```python
from build123d import *

# Parameters (mm, degrees)
SKETCH1_R           = 3.35
BOSS_EXTRUDE1_DEPTH = 300


with BuildPart() as part:
    # Sketch1 → Boss-Extrude1 (new body)
    with BuildSketch(Plane.XY):
        with BuildLine():
            Line((-9.853553391, -11.978553391), (-5.771446609, -7.896446609))
            ThreePointArc((-5.771446609, -7.896446609), (-5.609234935, -7.788060234), (-5.417893219, -7.75))
            Line((-5.417893219, -7.75), (5.417893219, -7.75))
            ThreePointArc((5.417893219, -7.75), (5.609234935, -7.788060234), (5.771446609, -7.896446609))
            Line((5.771446609, -7.896446609), (9.853553391, -11.978553391))
            ThreePointArc((9.853553391, -11.978553391), (9.961939766, -12.140765065), (10, -12.332106781))
            Line((10, -12.332106781), (10, -16))
            ThreePointArc((10, -16), (9.707106781, -16.707106781), (9, -17))
            Line((9, -17), (8, -17))
            ThreePointArc((8, -17), (7.292893219, -16.707106781), (7, -16))
            ThreePointArc((7, -16), (6.853553391, -15.646446609), (6.5, -15.5))
            Line((6.5, -15.5), (5, -15.5))
            ThreePointArc((5, -15.5), (4.292893219, -15.792893219), (4, -16.5))
            Line((4, -16.5), (4, -18.5))
            ThreePointArc((4, -18.5), (4.439339828, -19.560660172), (5.5, -20))
            Line((5.5, -20), (17, -20))
            ThreePointArc((17, -20), (19.121320344, -19.121320344), (20, -17))
            Line((20, -17), (20, -5.5))
            ThreePointArc((20, -5.5), (19.560660172, -4.439339828), (18.5, -4))
            Line((18.5, -4), (16.5, -4))
            ThreePointArc((16.5, -4), (15.792893219, -4.292893219), (15.5, -5))
            Line((15.5, -5), (15.5, -6.5))
            ThreePointArc((15.5, -6.5), (15.646446609, -6.853553391), (16, -7))
            ThreePointArc((16, -7), (16.707106781, -7.292893219), (17, -8))
            Line((17, -8), (17, -9))
            ThreePointArc((17, -9), (16.707106781, -9.707106781), (16, -10))
            Line((16, -10), (12.332106781, -10))
            ThreePointArc((12.332106781, -10), (12.140765065, -9.961939766), (11.978553391, -9.853553391))
            Line((11.978553391, -9.853553391), (7.896446609, -5.771446609))
            ThreePointArc((7.896446609, -5.771446609), (7.788060234, -5.609234935), (7.75, -5.417893219))
            Line((7.75, -5.417893219), (7.75, 5.417893219))
            ThreePointArc((7.75, 5.417893219), (7.788060234, 5.609234935), (7.896446609, 5.771446609))
            Line((7.896446609, 5.771446609), (11.978553391, 9.853553391))
            ThreePointArc((11.978553391, 9.853553391), (12.140765065, 9.961939766), (12.332106781, 10))
            Line((12.332106781, 10), (16, 10))
            ThreePointArc((16, 10), (16.707106781, 9.707106781), (17, 9))
            Line((17, 9), (17, 8))
            ThreePointArc((17, 8), (16.707106781, 7.292893219), (16, 7))
            ThreePointArc((16, 7), (15.646446609, 6.853553391), (15.5, 6.5))
            Line((15.5, 6.5), (15.5, 5))
            ThreePointArc((15.5, 5), (15.792893219, 4.292893219), (16.5, 4))
            Line((16.5, 4), (18.5, 4))
            ThreePointArc((18.5, 4), (19.560660172, 4.439339828), (20, 5.5))
            Line((20, 5.5), (20, 17))
            ThreePointArc((20, 17), (19.121320344, 19.121320344), (17, 20))
            Line((17, 20), (5.5, 20))
            ThreePointArc((5.5, 20), (4.439339828, 19.560660172), (4, 18.5))
            Line((4, 18.5), (4, 16.5))
            ThreePointArc((4, 16.5), (4.292893219, 15.792893219), (5, 15.5))
            Line((5, 15.5), (6.5, 15.5))
            ThreePointArc((6.5, 15.5), (6.853553391, 15.646446609), (7, 16))
            ThreePointArc((7, 16), (7.292893219, 16.707106781), (8, 17))
            Line((8, 17), (9, 17))
            ThreePointArc((9, 17), (9.707106781, 16.707106781), (10, 16))
            Line((10, 16), (10, 12.332106781))
            ThreePointArc((10, 12.332106781), (9.961939766, 12.140765065), (9.853553391, 11.978553391))
            Line((9.853553391, 11.978553391), (5.771446609, 7.896446609))
            ThreePointArc((5.771446609, 7.896446609), (5.609234935, 7.788060234), (5.417893219, 7.75))
            Line((5.417893219, 7.75), (-5.417893219, 7.75))
            ThreePointArc((-5.417893219, 7.75), (-5.609234935, 7.788060234), (-5.771446609, 7.896446609))
            Line((-5.771446609, 7.896446609), (-9.853553391, 11.978553391))
            ThreePointArc((-9.853553391, 11.978553391), (-9.961939766, 12.140765065), (-10, 12.332106781))
            Line((-10, 12.332106781), (-10, 16))
            ThreePointArc((-10, 16), (-9.707106781, 16.707106781), (-9, 17))
            Line((-9, 17), (-8, 17))
            ThreePointArc((-8, 17), (-7.292893219, 16.707106781), (-7, 16))
            ThreePointArc((-7, 16), (-6.853553391, 15.646446609), (-6.5, 15.5))
            Line((-6.5, 15.5), (-5, 15.5))
            ThreePointArc((-5, 15.5), (-4.292893219, 15.792893219), (-4, 16.5))
            Line((-4, 16.5), (-4, 18.5))
            ThreePointArc((-4, 18.5), (-4.439339828, 19.560660172), (-5.5, 20))
            Line((-5.5, 20), (-17, 20))
            ThreePointArc((-17, 20), (-19.121320344, 19.121320344), (-20, 17))
            Line((-20, 17), (-20, 5.5))
            ThreePointArc((-20, 5.5), (-19.560660172, 4.439339828), (-18.5, 4))
            Line((-18.5, 4), (-16.5, 4))
            ThreePointArc((-16.5, 4), (-15.792893219, 4.292893219), (-15.5, 5))
            Line((-15.5, 5), (-15.5, 6.5))
            ThreePointArc((-15.5, 6.5), (-15.646446609, 6.853553391), (-16, 7))
            ThreePointArc((-16, 7), (-16.707106781, 7.292893219), (-17, 8))
            Line((-17, 8), (-17, 9))
            ThreePointArc((-17, 9), (-16.707106781, 9.707106781), (-16, 10))
            Line((-16, 10), (-12.332106781, 10))
            ThreePointArc((-12.332106781, 10), (-12.140765065, 9.961939766), (-11.978553391, 9.853553391))
            Line((-11.978553391, 9.853553391), (-7.896446609, 5.771446609))
            ThreePointArc((-7.896446609, 5.771446609), (-7.788060234, 5.609234935), (-7.75, 5.417893219))
            Line((-7.75, 5.417893219), (-7.75, -5.417893219))
            ThreePointArc((-7.75, -5.417893219), (-7.788060234, -5.609234935), (-7.896446609, -5.771446609))
            Line((-7.896446609, -5.771446609), (-11.978553391, -9.853553391))
            ThreePointArc((-11.978553391, -9.853553391), (-12.140765065, -9.961939766), (-12.332106781, -10))
            Line((-12.332106781, -10), (-16, -10))
            ThreePointArc((-16, -10), (-16.707106781, -9.707106781), (-17, -9))
            Line((-17, -9), (-17, -8))
            ThreePointArc((-17, -8), (-16.707106781, -7.292893219), (-16, -7))
            ThreePointArc((-16, -7), (-15.646446609, -6.853553391), (-15.5, -6.5))
            Line((-15.5, -6.5), (-15.5, -5))
            ThreePointArc((-15.5, -5), (-15.792893219, -4.292893219), (-16.5, -4))
            Line((-16.5, -4), (-18.5, -4))
            ThreePointArc((-18.5, -4), (-19.560660172, -4.439339828), (-20, -5.5))
            Line((-20, -5.5), (-20, -17))
            ThreePointArc((-20, -17), (-19.121320344, -19.121320344), (-17, -20))
            Line((-17, -20), (-5.5, -20))
            ThreePointArc((-5.5, -20), (-4.439339828, -19.560660172), (-4, -18.5))
            Line((-4, -18.5), (-4, -16.5))
            ThreePointArc((-4, -16.5), (-4.292893219, -15.792893219), (-5, -15.5))
            Line((-5, -15.5), (-6.5, -15.5))
            ThreePointArc((-6.5, -15.5), (-6.853553391, -15.646446609), (-7, -16))
            ThreePointArc((-7, -16), (-7.292893219, -16.707106781), (-8, -17))
            Line((-8, -17), (-9, -17))
            ThreePointArc((-9, -17), (-9.707106781, -16.707106781), (-10, -16))
            Line((-10, -16), (-10, -12.332106781))
            ThreePointArc((-10, -12.332106781), (-9.961939766, -12.140765065), (-9.853553391, -11.978553391))
        make_face()
        Circle(SKETCH1_R, mode=Mode.SUBTRACT)
        with BuildLine():
            Line((-17, 11.78), (-13, 11.78))
            ThreePointArc((-13, 11.78), (-12.137329727, 12.137329727), (-11.78, 13))
            Line((-11.78, 13), (-11.78, 17))
            ThreePointArc((-11.78, 17), (-12.137329727, 17.862670273), (-13, 18.22))
            Line((-13, 18.22), (-17, 18.22))
            ThreePointArc((-17, 18.22), (-17.862670273, 17.862670273), (-18.22, 17))
            Line((-18.22, 17), (-18.22, 13))
            ThreePointArc((-18.22, 13), (-17.862670273, 12.137329727), (-17, 11.78))
        make_face(mode=Mode.SUBTRACT)
        with BuildLine():
            Line((-18.22, -13), (-18.22, -17))
            ThreePointArc((-18.22, -17), (-17.862670273, -17.862670273), (-17, -18.22))
            Line((-17, -18.22), (-13, -18.22))
            ThreePointArc((-13, -18.22), (-12.137329727, -17.862670273), (-11.78, -17))
            Line((-11.78, -17), (-11.78, -13))
            ThreePointArc((-11.78, -13), (-12.137329727, -12.137329727), (-13, -11.78))
            Line((-13, -11.78), (-17, -11.78))
            ThreePointArc((-17, -11.78), (-17.862670273, -12.137329727), (-18.22, -13))
        make_face(mode=Mode.SUBTRACT)
        with BuildLine():
            Line((13, -18.22), (17, -18.22))
            ThreePointArc((17, -18.22), (17.862670273, -17.862670273), (18.22, -17))
            Line((18.22, -17), (18.22, -13))
            ThreePointArc((18.22, -13), (17.862670273, -12.137329727), (17, -11.78))
            Line((17, -11.78), (13, -11.78))
            ThreePointArc((13, -11.78), (12.137329727, -12.137329727), (11.78, -13))
            Line((11.78, -13), (11.78, -17))
            ThreePointArc((11.78, -17), (12.137329727, -17.862670273), (13, -18.22))
        make_face(mode=Mode.SUBTRACT)
        with BuildLine():
            Line((18.22, 13), (18.22, 17))
            ThreePointArc((18.22, 17), (17.862670273, 17.862670273), (17, 18.22))
            Line((17, 18.22), (13, 18.22))
            ThreePointArc((13, 18.22), (12.137329727, 17.862670273), (11.78, 17))
            Line((11.78, 17), (11.78, 13))
            ThreePointArc((11.78, 13), (12.137329727, 12.137329727), (13, 11.78))
            Line((13, 11.78), (17, 11.78))
            ThreePointArc((17, 11.78), (17.862670273, 12.137329727), (18.22, 13))
        make_face(mode=Mode.SUBTRACT)
    extrude(amount=BOSS_EXTRUDE1_DEPTH)


solid = part.part
```
Can you work these out from the model? Positions are in its coordinate system, mm. A direction names the side the tool comes from. Give positions to 0.01 mm unless a question says otherwise; leave off trailing zeros. Loops run counter-clockwise (first coordinate to the right, second up) from the corner with the lowest first, then second, coordinate; pieces in that order, holes last. Notation, with made-up numbers: M 38.5,-36 L 97.5,-36 A18 cw 97.5,-25 Z; hole C -18.5,60 d5. An arc over 180 degrees is marked long. Use CSV: the item, a comma, the result in double quotes. Start each with the question number.
1. On a 3-axis mill with a long thin cutter (end or side, diameter ignored), from which of +Z, -Z, +X, -X, +Y, -Y can I reach the whole of each face in a straight line? I mean faces 1 (the face through (11, -20, 148)), 2 (the face through (-7.75, 0, 148)). Say none if no direction works.
2. For P1, Ø2, axis at x = -5.5, y = 4, coming from the -Z side; P2, Ø0.6, axis at y = -17.5, z = 133.5, coming from the +X side; P3, Ø1.6, axis at y = 18, z = 190, coming from the -X side; P4, Ø5, axis at x = 2, z = 203.5, coming from the -Y side, each with a flat end and sliding along its axis, tell me the tip position at first contact or that it passes through.
3. Imagine slicing it at C-C, the plane z = 116. Count the separate pieces of the cut face and the enclosed holes in it, plus the area to 3 significant figures.
4. If we mould it in two halves opening along X, with no side actions, what happens to faces 3 (the face through (-11, -20, 148)), 4 (the face through (20, 11, 148)), 5 (the face through (-3.347, 0.147, 147.9)), 6 (the face through (0, -7.75, 148))? For each: released by +X, released by -X, zero draft, split by the parting line, or undercut.
5. If I drill on L1, parallel to Y at x = 0, z = 221; L2, parallel to Y at x = 4.5, z = 271; L3, parallel to X at y = 13, z = 116.5, over which ranges is the centre line in solid material (lowest first)?
6. Imagine slicing it at A-A, the plane y = 0. Write out the boundary of the cut face in (x, z).
Response values:
1,face 1,"+Z, -Z, +X, -X, -Y"
1,face 2,"+Z, -Z"
2,P1,"z = 0"
2,P2,"x = 19.99"
2,P3,"x = -19.99"
2,P4,"y = -19.62"
3,separate pieces,"1"
3,enclosed holes,"5"
3,area,"670 mm^2"
4,face 3,"zero draft"
4,face 4,"released by +X"
4,face 5,"undercut"
4,face 6,"undercut"
5,L1,"-7.75 to -3.35, 3.35 to 7.75"
5,L2,"-19.62 to -15.63, -7.75 to 7.75, 15.63 to 19.62"
5,L3,"-20 to -18.22, -11.78 to -10, 10 to 11.78, 18.22 to 20"
6,outline,"M -7.75,0 L -3.35,0 L -3.35,300 L -7.75,300 Z; M 3.35,0 L 7.75,0 L 7.75,300 L 3.35,300 Z"
